Could you check a few things on this model? Use its own coordinates, in mm. A direction names the side the tool comes from. Coordinates: 2 decimals unless noted, no trailing zeros. Order: outer loops, then holes, each group sorted by start corner. A loop starts at its lowest first (then second) coordinate and runs counter-clockwise, first axis right, second up.
```python
from build123d import *

# Parameters (mm, degrees)
F0_R     = 50
F0_R_2   = 45
F1_DEPTH = 15
F2_W     = 30
F2_H     = 15
F3_DEPTH = 50
F5_W     = 30
F5_H     = 70
F5_W_2   = 28
F5_H_2   = 68
F6_DEPTH = 15
F7_W     = 28
F7_H     = 68
F8_DEPTH = 1


with BuildPart() as f1:
    # F0 (on Top) → F1 (new body)
    with BuildSketch(Plane.XY):
        Circle(F0_R)
        Circle(F0_R_2, mode=Mode.SUBTRACT)
    extrude(amount=F1_DEPTH)

    # F2 (on Front) → F3 (cut)
    with BuildSketch(Plane.XZ):
        with Locations((0, 7.5)):
            Rectangle(F2_W, F2_H)
    extrude(amount=F3_DEPTH, mode=Mode.SUBTRACT)

    # F5 (on face) → F6 (join)
    with BuildSketch(Plane.XY):
        with Locations((0, -26.421925)):
            Rectangle(F5_W, F5_H)
        with Locations((0, -26.421925)):
            Rectangle(F5_W_2, F5_H_2, mode=Mode.SUBTRACT)
    extrude(amount=F6_DEPTH)

    # F7 (on Top) → F8 (join)
    with BuildSketch(Plane.XY):
        with Locations((0, -26.421925)):
            Rectangle(F7_W, F7_H)
    extrude(amount=F8_DEPTH)


solid = f1.part
```
Item 1: Suppose I cut it at B-B (y = 0). List the corners of the cut face in (x, z) for me.
Item 2: I need wall thicknesses on line 1 (Y direction, x = -0.5, z = 13.5); line 2 (X direction, y = 0, z = 7.75); line 3 (X direction, y = -49.5, z = 11.25). Which ranges of each line are inside material? Lowest first, please.
Item 3: Suppose I cut it at C-C (z = 12). List the corners of the cut face in (x, y) for me.
Item 4: For pin 1 Ø2 at (y, z) = (-41.5, 8.5) entering from +X; pin 2 Ø4 at (x, z) = (-11.5, 11) entering from +Y; pin 3 Ø6 at (y, z) = (4, 3) entering from -X; pin 4 Ø8 at (x, y) = (-32.5, 22.5) entering from -Z, each with a flat end and sliding along its axis, tell me the tip position at first contact or that it passes through.
Item 5: Suppose I cut it at D-D (x = 38). List the corners of the cut face in (y, z) for me, and give its area (3 significant figures).
Item 6: Thinking about a two-plate mould opening in X: for faces 5 (the face through (1.99, 49.96, 7.4)), 6 (the face through (0, -61.422, 7)), 7 (the face through (14, -27, 8)), 8 (the face through (1.765, 44.965, 7.395)), which applies, +X half, -X half, draft (parallel to the pull), parting line (faces both ways), or undercut?
Item 7: Suppose I cut it at A-A (x = 0). List the corners of the cut face in (y, z) for me, and give its area (3 significant figures).
Item 8: Which directions (+Z, -Z, +X, -X, +Y, -Y) give clear straight access to the entire face, cutting with the end or side of a thin tool? Please do faces 1 (the face through (0, 7.578, 8)), 2 (the face through (15, -55, 7)), 3 (the face through (-15, -17, 7)), 4 (the face through (-15, -55, 7)).
Geometry results:
1. outline: (-50, 0) - (-45, 0) - (-45, 15) - (-50, 15) - close; (-15, 0) - (15, 0) - (15, 15) - (14, 15) - (14, 1) - (-14, 1) - (-14, 15) - (-15, 15) - close; (45, 0) - (50, 0) - (50, 15) - (45, 15) - close
2. line 1: y = -61.42 to -60.42, 7.58 to 8.58, 45 to 50
2. line 2: x = -50 to -45, -15 to -14, 14 to 15, 45 to 50
2. line 3: x = -15 to -14, 14 to 15
3. outline: (-15, -61.42) - (15, -61.42) - (15, -47.7) arc R50 ccw (long way) to (-15, -47.7) - close; hole (-15, -42.43) - (-15, 8.58) - (15, 8.58) - (15, -42.43) arc R45 ccw (long way) to start; hole (-14, -60.42) - (14, -60.42) - (14, 7.58) - (-14, 7.58) - close
4. pin 1: stops at x = 29.32
4. pin 2: stops at y = 49.09
4. pin 3: stops at x = -49.99
4. pin 4: passes through
5. outline: (-32.5, 0) - (-24.1, 0) - (-24.1, 15) - (-32.5, 15) - close; (24.1, 0) - (32.5, 0) - (32.5, 15) - (24.1, 15) - close
5. area: 252 mm2
6. face 5: parting line
6. face 6: draft
6. face 7: undercut
6. face 8: undercut
7. outline: (-61.42, 0) - (8.58, 0) - (8.58, 15) - (7.58, 15) - (7.58, 1) - (-60.42, 1) - (-60.42, 15) - (-61.42, 15) - close; (45, 0) - (50, 0) - (50, 15) - (45, 15) - close
7. area: 173 mm2
8. face 1: +Z
8. face 2: +Z, -Z, +X, -Y
8. face 3: +Z, -Z
8. face 4: +Z, -Z, -X, -Y
